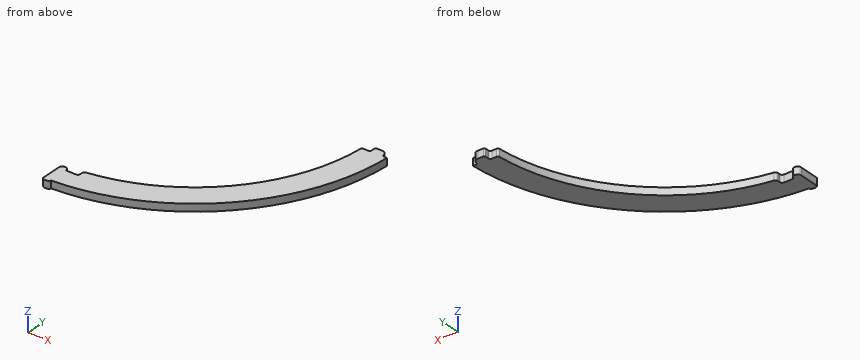
Autodesk Inventor part; units mm, degrees
ref_plane "YZ Plane" through (0, 0, 0) normal (1, 0, 0) x (0, 1, 0)
ref_plane "XZ Plane" through (0, 0, 0) normal (0, 1, 0) x (-1, 0, 0)
ref_plane "XY Plane" through (0, 0, 0) normal (0, 0, 1) x (1, 0, 0)
sketch "Sketch1" plane through (0, 0, 0) normal (0, 0, 1) x (1, 0, 0)
  arc A0 (2, -80.9753) -> (80.9861, -1.5) centre (0, 0) ccw
  arc A1 (10, -70.2922) -> (70.9842, -1.5) centre (0, 0) ccw
  line L0 (10, -73.0753) -> (10, -70.2922)
  line L1 (70.9842, -1.5) -> (80.9861, -1.5)
  line L2 (0, 0) -> (0, 0) construction
  line L3 (10, -73.0753) -> (2, -73.0753)
  line L4 (2, -73.0753) -> (2, -80.9753)
  point P0 (75.9851, -1.5)
  dimension "d0" = 162
  dimension "d1" = 142
  dimension "d12" = 8
  dimension "d13" = 2
  dimension "d14" = 7.9
  dimension "d23" = 1.5
extrude "Extrusion1" add sketch "Sketch1" along normal blind 3
sketch "Sketch3" plane through (0, 0, 3) normal (0, 0, 1) x (1, 0, 0)
  line L0 (10, -73.0753) -> (2, -73.0753)
  circle A0 centre (3.5, -73.0753) radius 1.5
  line L1 (2, -73.0753) -> (2, -80.9753) construction
  line L2 (2, -77.0253) -> (11.8753, -77.0253) construction
  ellipse E0 centre (3.5, -81.0253) end of major axis (5, -81.0253) minor radius 0.75
  point P0 (0, 0)
  point P1 (5, -73.0753)
  dimension "d15" = 3
  dimension "d16" = 1.5
  dimension "d20" = 0.75
  dimension "d21" = 1.5
  dimension "d22" = 4
extrude "Extrusion3" add sketch "Sketch3" against normal up to surface (3 mm away) contours L0 A0 | E0 picked at (3.784, -72.1991)
fillet "Fillet1" radius 1 2 edges at (10, -73.0753, 1.5) (10, -70.2922, 1.5)
sketch "Sketch4" plane through (0, 0, 3) normal (0, 0, 1) x (1, 0, 0)
  line L0 (80.9861, -1.5) -> (70.9842, -1.5)
  line L1 (80.9861, -1.5) -> (78.9861, -1.5)
  line L2 (78.9861, -4) -> (80.9012, -4)
  arc A0 (4.9576, -80.8481) -> (80.9861, -1.5) centre (0, 0) ccw
  arc A1 (80.9012, -4) -> (80.9861, -1.5) centre (0, 0) ccw
  line L3 (78.9861, -1.5) -> (78.9861, -4)
  line L4 (74.2542, -1.5) -> (70.9842, -1.5)
  arc A2 (10.8472, -70.1665) -> (70.9842, -1.5) centre (0, 0) ccw
  arc A3 (70.8727, -4.25) -> (70.9842, -1.5) centre (0, 0) ccw
  line L5 (70.8727, -4.25) -> (74.2542, -4.25)
  line L6 (74.2542, -4.25) -> (74.2542, -1.5)
  point P0 (10, -70.2922)
  dimension "d25" = 2.5
  dimension "d30" = 2
  dimension "d31" = 2.75
  dimension "d32" = 3.27
extrude "Extrusion4" cut sketch "Sketch4" against normal blind 10
fillet "Fillet3" radius 0.75 3 edges at (70.8727, -4.25, 1.5) (74.2542, -4.25, 1.5) (78.9861, -4, 1.5)
fillet "Fillet4" radius 2 1 edges at (78.9861, -1.5, 1.5)
fillet "Fillet5" radius 0.5 1 edges at (74.2542, -1.5, 1.5)
equation "\"d16\" = 0.5 * d15"
properties part number "shim_cartridge_V3"
Input: part model. Units: mm. Frame: model coordinates. Round coordinates to 2 decimals unless told otherwise and drop trailing zeros. Order: outer loops, then holes, each group sorted by start corner. A loop starts at its lowest first (then second) coordinate and runs counter-clockwise, first axis right, second up. Notation, with made-up numbers: (86, 52.25) - (131, 52.25) arc R31 cw to (131, 79.25) - close; hole circle Ø5 at (-26, 83.25). An arc over 180 degrees is marked (long way). One line per question, with ' | ' between items. Start each with the question number.
1) Ray query, probe 1 along X at (y, z) = (-70.5, 0.75); probe 2 along X at (y, z) = (-37, 0.4); probe 3 along Y at (x, z) = (13, 1.25). Return the intervals inside material, ascending.
2) Cut plane B-B, the plane y = -60. Return the cut outline in (x, z), then the cut area to 3 significant figures.
3) Cut plane A-A, the plane x = 45. Return the cut outline in (y, z).
4) Contact query for flat-ended pins moving along their axis: P1, Ø1.5, axis at x = 6, z = 1.5, coming from the +Y side; P2, Ø1.5, axis at y = -71, z = 1.5, coming from the -X side; P3, Ø1, axis at y = -50.5, z = 1, coming from the -X side. Output: stop coordinate, or through.
Worked out:
1) probe 1: x = 10.24 to 39.88 | probe 2: x = 60.6 to 72.06 | probe 3: y = -79.95 to -69.8
2) outline: (37.96, 0) - (54.42, 0) - (54.42, 3) - (37.96, 3) - close | area: 49.4 mm^2
3) outline: (-67.35, 0) - (-54.92, 0) - (-54.92, 3) - (-67.35, 3) - close
4) P1: stops at y = -73.08 | P2: stops at x = 2.8 | P3: stops at x = 49.4
